```python
from build123d import *

# Parameters (mm, degrees)
SKETCH1_R           = 9.35
SKETCH1_R_2         = 7.5
BOSS_EXTRUDE1_DEPTH = 34
FILLET1_R           = 2
SKETCH2_R           = 7.5
BOSS_EXTRUDE2_DEPTH = 34
SKETCH3_R           = 4.7
CUT_EXTRUDE1_DEPTH  = 40
CUT_EXTRUDE2_DEPTH  = 8.5
SKETCH5_W           = 14.5
SKETCH5_H           = 8.5
CUT_EXTRUDE3_DEPTH  = 10
CUT_EXTRUDE10_DEPTH = 10.5


with BuildPart() as part:
    # Sketch1 → Boss-Extrude1 (new body)
    with BuildSketch(Plane(origin=(0, 0, 0), x_dir=(1, 0, 0), z_dir=(0, 1, 0))):
        with Locations(Location((0, 0, 0), (0, 0, 270))):
            Circle(SKETCH1_R)
        with Locations(Location((0, 0, 0), (0, 0, 270))):
            Circle(SKETCH1_R_2, mode=Mode.SUBTRACT)
    extrude(amount=BOSS_EXTRUDE1_DEPTH)

    # Fillet1
    # the kernel refuses this fillet: 2 mm, written as the material it takes off along each edge
    with BuildSketch(Plane(origin=(0, 34, 0), x_dir=(0, 0, 1), z_dir=(-1, 0, 0))) as fillet1_piece_1:
        with BuildLine():
            CenterArc((7.35, -1.994367068), FILLET1_R, 0, 85.698777695)
            Line((7.5, 0), (7.503, 0.039887341))
            ThreePointArc((7.503, 0.039887341), (8.425, 0.04), (9.35, 0.04))
            Line((9.35, 0.04), (9.39, 0))
            Line((9.39, 0), (9.39, -1.994367068))
            Line((9.39, -1.994367068), (9.35, -1.994367068))
        make_face()
    revolve(axis=Axis((0, 34, 0), (0, 1, 0)), mode=Mode.SUBTRACT)

    # Sketch2 → Boss-Extrude2 (add)
    with BuildSketch(Plane(origin=(0, 0, 0), x_dir=(-1, 0, 0), z_dir=(0, -1, 0))):
        Circle(SKETCH2_R)
    extrude(amount=-BOSS_EXTRUDE2_DEPTH)

    # Sketch3 → Cut-Extrude1 (cut)
    with BuildSketch(Plane(origin=(0, 0, 0), x_dir=(-1, 0, 0), z_dir=(0, -1, 0))):
        with Locations(Location((0, 0, 0), (0, 0, 90))):
            Circle(SKETCH3_R)
    extrude(amount=-CUT_EXTRUDE1_DEPTH, mode=Mode.SUBTRACT)

    # Sketch4 → Cut-Extrude2 (cut)
    with BuildSketch(Plane(origin=(0, 11, 0), x_dir=(1, 0, 0), z_dir=(0, 1, 0))):
        Polygon((0, -8.371578903), (7.25, -4.185789452), (7.25, 4.185789452), (0, 8.371578903), (-7.25, 4.185789452), (-7.25, -4.185789452), align=None)
    extrude(amount=-CUT_EXTRUDE2_DEPTH, mode=Mode.SUBTRACT)

    # Sketch5 → Cut-Extrude3 (cut)
    with BuildSketch(Plane.XY):
        with Locations((0, 6.75)):
            Rectangle(SKETCH5_W, SKETCH5_H)
    extrude(amount=-CUT_EXTRUDE3_DEPTH, mode=Mode.SUBTRACT)

    # Sketch6 → Cut-Extrude10 (cut)
    with BuildSketch(Plane(origin=(0, 17, 0), x_dir=(1, 0, 0), z_dir=(0, 1, 0))):
        Polygon((-7.25, 4.185789452), (-7.25, -4.185789452), (-7.25, -13.840874754), (7.25, -13.840874754), (7.25, -4.185789452), (7.25, 4.185789452), align=None)
        Polygon((7.25, 4.185789452), (-7.25, 4.185789452), (0, 8.371578903), align=None)
    extrude(amount=CUT_EXTRUDE10_DEPTH, mode=Mode.SUBTRACT)


solid = part.part
```
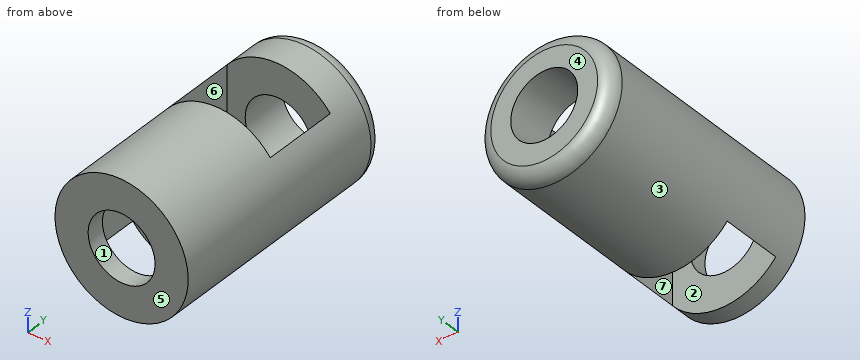
Source: CAD feature listing. Evaluate the final solid. Frame: model axes, mm. Face numbers are marked on the shaded views. A direction names the side the tool comes from. Coordinates: 2 decimals unless noted, no trailing zeros. Order: outer loops, then holes, each group sorted by start corner. A loop starts at its lowest first (then second) coordinate and runs counter-clockwise, first axis right, second up. Notation, with made-up numbers: M -6.75,51.5 L 17.25,51.5 A18 cw 17.25,62.5 Z; hole C 46.5,59.25 d5. An arc over 180 degrees is marked long. Write each question's results on one line, items separated by ' | '. Start each with the question number.
1) Draft query along X for the marked faces 1, 2, 3 and 4. Return one class per face: released by +X, released by -X, zero draft, split by the parting line, or undercut.
2) Section query C-C (x = -3.5). Give the number of separate pieces and of enclosed holes in the cut face, plus the area to 3 significant figures.
3) Contact query for flat-ended pins moving along their axis: pin 1 Ø9.5 at (y, z) = (8, 0.5) entering from +X; pin 2 Ø4 at (y, z) = (4.5, -3) entering from -X; pin 3 Ø1.5 at (x, y) = (-3.5, 15.5) entering from +Z; pin 4 Ø3 at (y, z) = (29, -5) entering from +X. Output: stop coordinate, or through.
4) Section query B-B (y = 22.5). Return the cut outline in (x, z), plus the area to 3 significant figures.
5) Line query: line 1 (Y direction, x = -4.5, z = -4); line 2 (X direction, y = 31, z = 0). Output: solid intervals per line, ascending. Write a range as from..to.
6) Access query for the marked faces 5, 6 and 7. Directions: +Z, -Z, +X, -X, +Y, -Y. A direction counts if a zero-diameter tool reaches every point of the face in a straight line with its end or side. Return the directions, or none.
7) Section query A-A (z = 0). Return the cut outline in (x, y).
Answers:
1) face 1: undercut | face 2: undercut | face 3: split by the parting line | face 4: zero draft
2) separate pieces: 4 | enclosed holes: 0 | area: 208 mm^2
3) pin 1: stops at x = 9.35 | pin 2: stops at x = -9.3 | pin 3: stops at z = 8.94 | pin 4: stops at x = 8.67
4) outline: M -7.25,-4.19 L -7.25,5.9 A9.35 ccw long 7.25,5.9 L 7.25,-4.19 L 0,-8.37 Z | area: 63.2 mm^2
5) line 1: y = 0..2.5, 11..17, 27.5..34 | line 2: x = -9.35..-4.7, 4.7..9.35
6) face 5: +Z, -Z, +X, -X, -Y | face 6: +Z | face 7: -Z
7) outline: M -9.35,0 L -4.7,0 L -4.7,2.5 L -7.25,2.5 L -7.25,11 L -4.7,11 L -4.7,17 L -7.25,17 L -7.25,27.5 L -4.7,27.5 L -4.7,34 L -7.5,34 A2 ccw -9.35,32.01 Z; M 4.7,0 L 9.35,0 L 9.35,32.01 A2 ccw 7.5,34 L 4.7,34 L 4.7,27.5 L 7.25,27.5 L 7.25,17 L 4.7,17 L 4.7,11 L 7.25,11 L 7.25,2.5 L 4.7,2.5 Z
